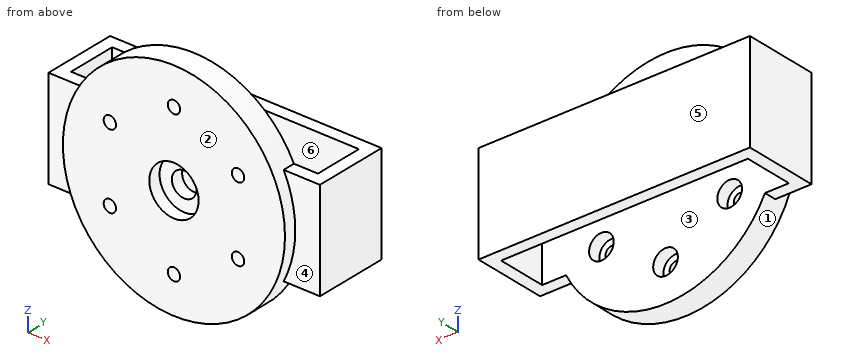
```python
from build123d import *

# Parameters (mm, degrees)
SKETCH1_R                = 45
SKETCH1_R_2              = 2.5
SKETCH1_R_3              = 10
BOSS_EXTRUDE1_DEPTH      = 10
SKETCH2_W                = 110
SKETCH2_H                = 40
BOSS_EXTRUDE2_DEPTH      = 25
BOSS_EXTRUDE2_DEPTH_BACK = 5
SKETCH3_W                = 100
SKETCH3_H                = 20
CUT_EXTRUDE1_DEPTH       = 45
SKETCH4_R                = 5
CUT_EXTRUDE2_DEPTH       = 5


with BuildPart() as part:
    # Sketch1 → Boss-Extrude1 (new body)
    with BuildSketch(Plane(origin=(0, 0, 0), x_dir=(1, 0, 0), z_dir=(0, 1, 0))):
        Circle(SKETCH1_R)
        with Locations((0, 30)):
            Circle(SKETCH1_R_2, mode=Mode.SUBTRACT)
        with Locations((25.980762114, 15)):
            Circle(SKETCH1_R_2, mode=Mode.SUBTRACT)
        with Locations((25.980762114, -15)):
            Circle(SKETCH1_R_2, mode=Mode.SUBTRACT)
        with Locations((0, -30)):
            Circle(SKETCH1_R_2, mode=Mode.SUBTRACT)
        with Locations((-25.980762114, -15)):
            Circle(SKETCH1_R_2, mode=Mode.SUBTRACT)
        with Locations((-25.980762114, 15)):
            Circle(SKETCH1_R_2, mode=Mode.SUBTRACT)
        Circle(SKETCH1_R_3, mode=Mode.SUBTRACT)
    extrude(amount=BOSS_EXTRUDE1_DEPTH)

    # Sketch2 → Boss-Extrude2 (add, two sides)
    with BuildSketch(Plane(origin=(0, 10, 0), x_dir=(1, 0, 0), z_dir=(0, 1, 0))) as boss_extrude2_sk:
        Rectangle(SKETCH2_W, SKETCH2_H)
    extrude(amount=BOSS_EXTRUDE2_DEPTH)
    extrude(boss_extrude2_sk.sketch, amount=-BOSS_EXTRUDE2_DEPTH_BACK)

    # Sketch3 → Cut-Extrude1 (cut)
    with BuildSketch(Plane(origin=(0, 0, -20), x_dir=(-1, 0, 0), z_dir=(0, 0, -1))):
        with Locations((0, 20)):
            Rectangle(SKETCH3_W, SKETCH3_H)
    extrude(amount=-CUT_EXTRUDE1_DEPTH, mode=Mode.SUBTRACT)

    # Sketch4 → Cut-Extrude2 (cut)
    with BuildSketch(Plane(origin=(0, 10, 0), x_dir=(1, 0, 0), z_dir=(0, 1, 0))):
        with Locations((0, 30)):
            Circle(SKETCH4_R)
        with Locations((25.980762114, 15)):
            Circle(SKETCH4_R)
        with Locations((25.980762114, -15)):
            Circle(SKETCH4_R)
        with Locations((0, -30)):
            Circle(SKETCH4_R)
        with Locations((-25.980762114, -15)):
            Circle(SKETCH4_R)
        with Locations((-25.980762114, 15)):
            Circle(SKETCH4_R)
        Circle(SKETCH4_R)
    extrude(amount=-CUT_EXTRUDE2_DEPTH, mode=Mode.SUBTRACT)


solid = part.part
```
Source: CAD feature listing. Evaluate the final solid. Frame: model axes, mm. Face numbers are marked on the shaded views. A direction names the side the tool comes from. Coordinates: 2 decimals unless noted, no trailing zeros. Loops run counter-clockwise (first coordinate to the right, second up) from the corner with the lowest first, then second, coordinate; pieces in that order, holes last. Notation, with made-up numbers: (89, 37) -> (100, 37) arc R29 ccw to (100, 69) -> close; hole circle Ø3 at (70.5, 38.5). An arc over 180 degrees is marked (long way). One line per item, written item: value. Start each with the question number.
Q1. Set-up query: the marked faces 1, 2 and 3. Return all of +Z, -Z, +X, -X, +Y, -Y with unobstructed straight access to the full face (end or side cutting, diameter ignored); none if empty.
Q2. Section query D-D, the plane z = 0. Return the cut outline in (x, y).
Q3. Section query B-B, the plane x = 0. Give the number of separate pieces and of enclosed holes in the cut face, and give its area (3 significant figures).
Q4. Section query A-A, the plane y = 18. Return the cut outline in (x, z).
Q5. Mould query, pull axis Y, two halves, no side actions, for the marked faces 4, 5 and 6. Classes: pulls with the +Y half, pulls with the -Y half, needs draft (parallel to the pull), parting line crosses it, or undercut.
Q6. Contact query for flat-ended pins moving along their axis: P1, Ø4, axis at x = 32, z = -32, coming from the +Y side; P2, Ø6, axis at x = 12, y = 24.5, coming from the -Z side; P3, Ø6, axis at x = 0, z = 0, coming from the -Y side; P4, Ø6, axis at x = -4, z = -1, coming from the -Y side. Output: stop coordinate, or through.
Q7. Line query: line 1 along Z through (x, y) = (0, 2.5); line 2 along X through (y, z) = (6.5, -14.5); line 3 along Z through (x, y) = (0, 6.15). Output: solid intervals per line, ascending.
Q8. Section query C-C, the plane z = -15. Return the cut outline in (x, y).
Results:
1. face 1: -Y
1. face 2: +Z, -Z, +X, -X, -Y
1. face 3: +Z, -Z
2. outline: (-55, 5) -> (-45, 5) -> (-45, 0) -> (-10, 0) -> (-10, 5) -> (-5, 5) -> (-5, 10) -> (-50, 10) -> (-50, 30) -> (50, 30) -> (50, 10) -> (5, 10) -> (5, 5) -> (10, 5) -> (10, 0) -> (45, 0) -> (45, 5) -> (55, 5) -> (55, 35) -> (-55, 35) -> close
3. separate pieces: 5
3. enclosed holes: 0
3. area: 800 mm^2
4. outline: (-55, -20) -> (-50, -20) -> (-50, 20) -> (-55, 20) -> close; (50, -20) -> (55, -20) -> (55, 20) -> (50, 20) -> close
5. face 4: pulls with the -Y half
5. face 5: pulls with the +Y half
5. face 6: undercut
6. P1: y = 10
6. P2: through
6. P3: y = 30
6. P4: y = 5
7. line 1: -45 to -32.5, -27.5 to -10, 10 to 27.5, 32.5 to 45
7. line 2: -55 to -30.96, -21.01 to 21.01, 30.96 to 55
7. line 3: -45 to -35, -25 to -5, 5 to 25, 35 to 45
8. outline: (-55, 5) -> (-42.43, 5) -> (-42.43, 0) -> (-28.48, 0) -> (-28.48, 5) -> (-30.98, 5) -> (-30.98, 10) -> (-50, 10) -> (-50, 30) -> (50, 30) -> (50, 10) -> (30.98, 10) -> (30.98, 5) -> (28.48, 5) -> (28.48, 0) -> (42.43, 0) -> (42.43, 5) -> (55, 5) -> (55, 35) -> (-55, 35) -> close; (-23.48, 0) -> (23.48, 0) -> (23.48, 5) -> (20.98, 5) -> (20.98, 10) -> (-20.98, 10) -> (-20.98, 5) -> (-23.48, 5) -> close
